from build123d import *

# Parameters (mm, degrees)
SKETCH1_W                = 100
SKETCH1_H                = 100
BOSS_EXTRUDE1_DEPTH      = 1400
BOSS_EXTRUDE3_DEPTH      = 400
BOSS_EXTRUDE3_DEPTH_BACK = 200
SKETCH3_R                = 15
SKETCH4_R                = 40
BOSS_EXTRUDE4_DEPTH      = 10
BOSS_EXTRUDE5_START      = 250
SKETCH5_R                = 40
BOSS_EXTRUDE5_DEPTH      = 250


with BuildPart() as part:
    # Sketch1 → Boss-Extrude1 (new body)
    with BuildSketch(Plane.XY):
        Rectangle(SKETCH1_W, SKETCH1_H)
    extrude(amount=BOSS_EXTRUDE1_DEPTH)

    # Sketch3 → Boss-Extrude3 (add, two sides: drawn at the far end of the back side and taken through both)
    with BuildSketch(Plane.XZ.offset(50).offset(-BOSS_EXTRUDE3_DEPTH_BACK)):
        with Locations((0, 700)):
            Circle(SKETCH3_R)
    extrude(amount=BOSS_EXTRUDE3_DEPTH + BOSS_EXTRUDE3_DEPTH_BACK)

    # Sketch4 → Boss-Extrude4 (add)
    with BuildSketch(Plane.XZ.offset(450)):
        with Locations((0, 700)):
            Circle(SKETCH4_R)
    extrude(amount=-BOSS_EXTRUDE4_DEPTH)

    # Sketch5 → Boss-Extrude5 (add)
    with BuildSketch(Plane.XZ.offset(50).offset(BOSS_EXTRUDE5_START)):
        with Locations(Location((0, 700, 0), (0, 0, 180))):
            Circle(SKETCH5_R)
    extrude(amount=-BOSS_EXTRUDE5_DEPTH)


solid = part.part
CAD build for the part. Positions are in the model's coordinates, mm. A direction names the side the tool comes from. Round coordinates to 2 decimals unless told otherwise and drop trailing zeros. Loops run counter-clockwise (first coordinate to the right, second up) from the corner with the lowest first, then second, coordinate; pieces in that order, holes last.
(1) Which spindle directions (+Z, -Z, +X, -X, +Y, -Y) get a long thin tool onto all of the face, cutting with end or side? Do faces 5 (the cylindrical face through (8.67, -176.75, 739.05)), 6 (the cylindrical face through (-3.252, 100.7, 685.357)), 7 (the flat face through (17, -440, 701)). Say none if no direction does.
(2) Cut at C-C (y = -388). Give the cut face in (x, z).
(3) Wall check: line 1 along Y through (x, z) = (40, 977); line 2 along Z through (x, y) = (2, -166.5); line 3 along Z through (x, y) = (32, -133). Give the ranges that are in metal, low to high.
(4) Cut at B-B (z = 700). Give the cut face in (x, y).
(5) Two-plate mould, pull along Y, no slides. Class faces 1 (the flat face through (-17, -300, 699)), 2 (the flat face through (-45, -50, 690)), 3 (the flat face through (-12, 50, 690)), 4 (the flat face through (-1, 1, 1400)): +Y half, -Y half, draft (parallel to the pull), parting line (faces both ways), or undercut.
(6) Cut at A-A (x = 0). Give the cut face in (y, z), plus the area to 3 significant figures.
(7) Cut at D-D (z = 497.5). Give the cut face in (x, y), plus the area to 3 significant figures.
(8) Drop flat-ended pins along their axis: pin 1 (1.5 mm diameter, centred on x = -10.5, y = -377.5, fed in from +Z); pin 2 (3 mm diameter, centred on x = -15.5, z = 1251, fed in from -Y); pin 3 (4 mm diameter, centred on x = 28, z = 773, fed in from +Y). Give the stop position or say it passes through.
Findings below:
1. face 5: -Y
1. face 6: +Y
1. face 7: none
2. outline: circle Ø30 at (0, 700)
3. line 1: y = -50 to 50
3. line 2: z = 660.05 to 739.95
3. line 3: z = 676 to 724
4. outline: (-50, -50) - (-40, -50) - (-40, -300) - (-15, -300) - (-15, -440) - (-40, -440) - (-40, -450) - (40, -450) - (40, -440) - (15, -440) - (15, -300) - (40, -300) - (40, -50) - (50, -50) - (50, 50) - (15, 50) - (15, 150) - (-15, 150) - (-15, 50) - (-50, 50) - close
5. face 1: undercut
5. face 2: -Y half
5. face 3: +Y half
5. face 4: draft
6. outline: (-450, 660) - (-440, 660) - (-440, 685) - (-300, 685) - (-300, 660) - (-50, 660) - (-50, 0) - (50, 0) - (50, 685) - (150, 685) - (150, 715) - (50, 715) - (50, 1400) - (-50, 1400) - (-50, 740) - (-300, 740) - (-300, 715) - (-440, 715) - (-440, 740) - (-450, 740) - close
6. area: 168,000 mm2
7. outline: (-50, -50) - (50, -50) - (50, 50) - (-50, 50) - close
7. area: 10,000 mm2
8. pin 1: stops at z = 711.4
8. pin 2: stops at y = -50
8. pin 3: stops at y = 50
